Could you check a few things on this model? Use its own coordinates, in mm. Face numbers are marked on the shaded views. Coordinates: 2 decimals unless noted, no trailing zeros. Order: outer loops, then holes, each group sorted by start corner. A loop starts at its lowest first (then second) coordinate and runs counter-clockwise, first axis right, second up. Notation, with made-up numbers: (-37.5, 44.25) -> (2.5, 44.25) arc R25 cw to (2.5, 58.25) -> close; hole circle Ø8 at (17.25, 34.25). An arc over 180 degrees is marked (long way). Use a Markdown table: item, result. Add a question column.
1) If I drill on L1, parallel to X at y = 68, z = 100.5; L2, parallel to Y at x = 29.5, z = 11; L3, parallel to Y at x = 52, z = 28.5, over which ranges is the centre line in solid material (lowest first)? Write a range as [from, to].
2) If we section it at A-A (z = 98.5): Write out the boundary of the cut face in (x, y).
3) If we section it at D-D (y = 68.5): Write out the boundary of the cut face in (x, z).
4) Thinking about a two-plate mould opening in X: for the marked faces 1, 2, 3 and 4, which applies, +X half, -X half, draft (parallel to the pull), parting line (faces both ways), or undercut?
5) If we section it at C-C (z = 85.5): Write out the boundary of the cut face in (x, y).
6) If we section it at B-B (y = 12): Write out the boundary of the cut face in (x, z).
7) Will these pins go through, and if not, where does the flat tip stop? pin 1 Ø4 at (y, z) = (46.5, 46.5) entering from +X; pin 2 Ø6 at (y, z) = (58.48, 57.68) entering from -X; pin 3 Ø9.5 at (x, z) = (17.03, 37.15) entering from +Y; pin 4 Ø2 at (y, z) = (19.5, 53.5) entering from +X.
Autodesk Inventor part; units mm, degrees
ref_plane "Work Plane1" through (17.0319, 0, 117.3988) normal (1, 0, 0) x (0, 1, 0)
ref_plane "YZ Plane" through (0, 0, 0) normal (1, 0, 0) x (0, 1, 0)
ref_plane "XZ Plane" through (0, 0, 0) normal (0, 1, 0) x (-1, 0, 0)
sketch "Sketch1" plane through (0, 0, 0) normal (0, 0, 1) x (1, 0, 0)
  line L0 (-26.1481, 3.048) -> (60.2119, 3.048)
  line L1 (60.2119, 3.048) -> (60.2119, 0)
  line L2 (60.2119, 0) -> (-26.1481, 0)
  line L3 (-26.1481, 0) -> (-26.1481, 3.048)
  line L4 (-26.1481, 0) -> (-23.1001, 0)
  line L5 (-23.1001, 0) -> (-23.1001, 78.613)
  line L6 (-23.1001, 78.613) -> (-26.1481, 78.613)
  line L7 (-26.1481, 78.613) -> (-26.1481, 0)
  line L8 (60.2119, 0) -> (57.1639, 0)
  line L9 (57.1639, 0) -> (57.1639, 78.613)
  line L10 (57.1639, 78.613) -> (60.2119, 78.613)
  line L11 (60.2119, 78.613) -> (60.2119, 0)
  point P0 (0, 0)
  dimension "d0" = 86.36
  dimension "d1" = 3.048
  dimension "d2" = 3.048
  dimension "d3" = 3.048
  dimension "d4" = 78.613
  dimension "d5" = 0
extrude "Extrusion1" add sketch "Sketch1" along normal blind 123.7488
fillet "Fillet1" radius 12.7 2 edges at (58.6879, 78.613, 123.7488) (-24.6241, 78.613, 123.7488)
sketch "Sketch2" plane through (60.2119, 0, 0) normal (1, 0, 0) x (0, 0, -1)
  arc A0 (-111.0488, 78.613) -> (-123.7488, 65.913) centre (-111.0488, 65.913) ccw
  circle A1 centre (-111.0488, 65.913) radius 4.7625
  dimension "d9" = 9.525
extrude "Extrusion2" cut sketch "Sketch2" against normal through all
fillet "Fillet2" radius 6.35 4 edges at (57.1639, 3.048, 61.8744) (60.2119, 0, 61.8744) (-23.1001, 3.048, 61.8744) (-26.1481, 0, 61.8744)
sketch "Sketch3" plane through (60.2119, 78.613, 111.0488) normal (1, 0, 0) x (0, 0, -1)
  line L0 (111.0488, -72.263) -> (-12.7, -72.263)
  line L1 (111.0488, -72.263) -> (111.0488, 0)
  line L2 (111.0488, 0) -> (0, 0)
  line L3 (-12.7, -12.7) -> (-12.7, -72.263)
  line L4 (111.0488, -65.913) -> (-12.7, -65.913)
  line L5 (0, 0) -> (87.5082, -15.4301)
  line L6 (87.5082, -15.4301) -> (111.0488, -65.913)
  point P0 (111.0488, -78.613)
  dimension "d13" = 6.35
  dimension "d15" = 125
  dimension "d16" = 65
extrude "Extrusion3" cut sketch "Sketch3" against normal through all contours L6 L5 L2 L1
fillet "Fillet3" radius 12.7 2 edges at (58.6879, 63.1829, 23.5406) (-24.6241, 63.1829, 23.5406)
fillet "Fillet4" radius 12.7 2 edges at (58.6879, 12.7, 0) (-24.6241, 12.7, 0)
sketch "Sketch4" plane through (-16.7501, 3.048, 0) normal (0, 1, 0) x (1, 0, 0)
  line L0 (0, -123.7488) -> (67.564, -123.7488)
  line L1 (67.564, 0) -> (0, 0)
  circle A0 centre (33.782, -11.7475) radius 5.3975
  circle A1 centre (33.782, -37.1475) radius 5.3975
  arc A2 (28.3845, -112.002) -> (39.1795, -112.002) centre (33.782, -112.0013) ccw
  arc A3 (39.1833, -81.0902) -> (28.3807, -81.0902) centre (33.782, -81.0895) ccw
  line L2 (28.3845, -112.002) -> (28.3807, -81.0902)
  line L3 (39.1833, -81.0902) -> (39.1795, -112.002)
  point P0 (16.7501, 0)
  dimension "d21" = 10.795
  dimension "d22" = 10.795
  dimension "d23" = 25.4
  dimension "d24" = 11.7475
  dimension "d25" = 10.795
  dimension "d26" = 10.8026
  dimension "d27" = 11.7475
  dimension "d28" = 30.9118
  dimension "d29" = 30.9118
  dimension "d30" = 30.9118
extrude "Extrusion4" cut sketch "Sketch4" against normal through all
sketch "Sketch5" plane through (60.2119, 6.35, 123.7488) normal (1, 0, 0) x (0, 0, -1)
  circle A0 centre (12.7, 59.563) radius 4.7625
  circle A1 centre (66.064, 25.146) radius 9.525
  circle A2 centre (66.064, 25.146) radius 11.43
  line L0 (0, -6.35) -> (123.7488, -6.35)
  dimension "d33" = 19.05
  dimension "d36" = 22.86
  dimension "d37" = 31.496
  dimension "d38" = 63.5
extrude "Extrusion5" add sketch "Sketch5" along normal blind 5.461 contours A2
sketch "Sketch6" plane through (60.2119, 31.496, 57.6848) normal (1, 0, 0) x (0, 0, -1)
  circle A0 centre (0, 0) radius 9.525
  point P0 (57.6848, -31.496)
ref_plane "Work Plane1" through (17.0319, 0, 117.3988) normal (1, 0, 0) x (0, 1, 0)
mirror "Mirror1" about plane through (17.0319, 0, 117.3988) normal (1, 0, 0) of "Extrusion5"
extrude "Extrusion6" cut sketch "Sketch6" against normal through all
fillet "Fillet5" radius 2.54 2 edges at (60.2119, 31.496, 69.1148) (-26.1482, 31.496, 69.1148)
sketch "Sketch7" plane through (60.2119, 6.35, 123.7488) normal (1, 0, 0) x (0, 0, -1)
  circle A0 centre (39.0765, 25.1459) radius 2.317
  circle A1 centre (93.0515, 25.1461) radius 2.317
  circle A2 centre (66.064, 25.146) radius 14.2875
  line L0 (97.8141, -6.6039) -> (97.814, 56.8961)
  line L1 (34.3141, -6.6041) -> (97.8141, -6.6039)
  line L2 (34.314, 56.8959) -> (34.3141, -6.6041)
  line L3 (97.814, 56.8961) -> (34.314, 56.8959)
  circle A3 centre (66.0641, -1.8415) radius 2.317
  circle A4 centre (66.064, 52.1335) radius 2.317
  point P0 (123.7488, -6.35)
extrude "Extrusion7" cut sketch "Sketch7" against normal up to surface (3.048 mm away) contours A0 | A1 | A4
equation "\"d27\" = d24"
equation "\"d29\" = d28"
properties part number "Ratchet Frame 1764"
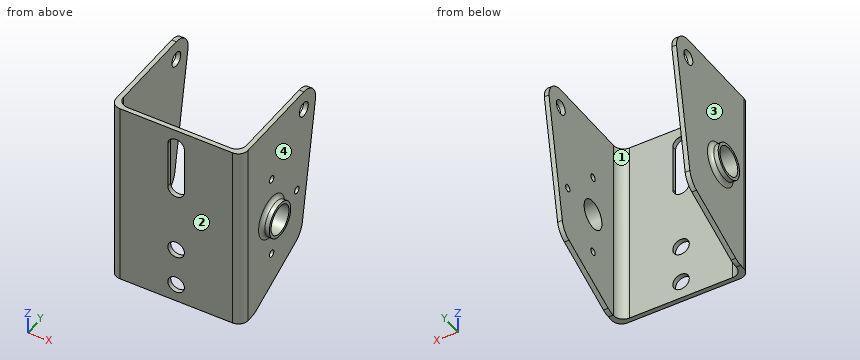
Answer sheet:
| question | item | result |
|---|---|---|
| 1 | L1 | [-26.15, -23.1], [57.16, 60.21] |
| 1 | L2 | [0, 3.05] |
| 1 | L3 | [0, 3.16] |
| 2 | outline | (-26.15, 6.35) arc R6.35 ccw to (-19.8, 0) -> (11.63, 0) -> (11.63, 3.05) -> (-16.75, 3.05) arc R6.35 cw to (-23.1, 9.4) -> (-23.1, 76.4) -> (-26.15, 76.4) -> close; (22.43, 0) -> (53.86, 0) arc R6.35 ccw to (60.21, 6.35) -> (60.21, 76.4) -> (57.16, 76.4) -> (57.16, 9.4) arc R6.35 cw to (50.81, 3.05) -> (22.43, 3.05) -> close |
| 3 | outline | (-26.15, 53.7) -> (-23.1, 53.7) -> (-23.1, 107.05) -> (-26.15, 107.05) -> close; (-26.15, 115.05) -> (-23.1, 115.05) -> (-23.1, 123.48) -> (-26.15, 123.48) -> close; (57.16, 53.7) -> (60.21, 53.7) -> (60.21, 107.05) -> (57.16, 107.05) -> close; (57.16, 115.05) -> (60.21, 115.05) -> (60.21, 123.48) -> (57.16, 123.48) -> close |
| 4 | face 1 | undercut |
| 4 | face 2 | draft |
| 4 | face 3 | -X half |
| 4 | face 4 | +X half |
| 5 | outline | (-26.15, 6.35) arc R6.35 ccw to (-19.8, 0) -> (11.63, 0) -> (11.63, 3.05) -> (-16.75, 3.05) arc R6.35 cw to (-23.1, 9.4) -> (-23.1, 74.11) -> (-26.15, 74.11) -> close; (22.43, 0) -> (53.86, 0) arc R6.35 ccw to (60.21, 6.35) -> (60.21, 29.33) -> (57.16, 29.33) -> (57.16, 9.4) arc R6.35 cw to (50.81, 3.05) -> (22.43, 3.05) -> close; (57.16, 33.66) -> (60.21, 33.66) -> (60.21, 74.11) -> (57.16, 74.11) -> close |
| 6 | outline | (-26.15, 0.18) -> (-23.1, 0.18) -> (-23.1, 123.75) -> (-26.15, 123.75) -> close; (57.16, 0.18) -> (60.21, 0.18) -> (60.21, 123.75) -> (57.16, 123.75) -> close |
| 7 | pin 1 | x = 60.21 |
| 7 | pin 2 | x = -26.15 |
| 7 | pin 3 | through |
| 7 | pin 4 | x = 61.6 |
